```python
from build123d import *

# Parameters (mm, degrees)
SKETCH_1_W        = 30
SKETCH_1_H        = 30
SKETCH_1_W_2      = 26
SKETCH_1_H_2      = 26
EXTRUDE_1_DEPTH   = 270
EXTRUDE_1_2_DEPTH = 270
EXTRUDE_1_3_DEPTH = 270
EXTRUDE_1_4_DEPTH = 270
EXTRUDE_1_5_DEPTH = 270
EXTRUDE_1_6_DEPTH = 270
SKETCH_1_4_W      = 400
SKETCH_1_4_H      = 355
EXTRUDE_2_DEPTH   = 2
SKETCH_3_W        = 25
SKETCH_3_H        = 25
SKETCH_3_W_2      = 22
SKETCH_3_H_2      = 22
EXTRUDE_3_DEPTH   = 200
SKETCH_9_W        = 30
SKETCH_9_H        = 30
EXTRUDE_4_DEPTH   = 290
SKETCH_10_W       = 30
SKETCH_10_H       = 30
EXTRUDE_5_DEPTH   = 330


with BuildPart() as part:
    # Sketch 1 → Extrude 1 (new body)
    with BuildSketch(Plane.XY):
        with Locations((-139.865693992, 17.660065035)):
            Rectangle(SKETCH_1_W, SKETCH_1_H)
        with Locations((-139.865693992, 17.660065035)):
            Rectangle(SKETCH_1_W_2, SKETCH_1_H_2, mode=Mode.SUBTRACT)
    extrude(amount=EXTRUDE_1_DEPTH)



with BuildPart() as body_2:
    # Sketch 1 → Extrude 1 2 (new body)
    with BuildSketch(Plane.XY):
        with Locations((40.134306008, 17.660065035)):
            Rectangle(SKETCH_1_W, SKETCH_1_H)
        with Locations((40.134306008, 17.660065035)):
            Rectangle(SKETCH_1_W_2, SKETCH_1_H_2, mode=Mode.SUBTRACT)
    extrude(amount=EXTRUDE_1_2_DEPTH)


with BuildPart() as body_3:
    # Sketch 1 → Extrude 1 3 (new body)
    with BuildSketch(Plane.XY):
        with Locations((220.134306008, 17.660065035)):
            Rectangle(SKETCH_1_W, SKETCH_1_H)
        with Locations((220.134306008, 17.660065035)):
            Rectangle(SKETCH_1_W_2, SKETCH_1_H_2, mode=Mode.SUBTRACT)
    extrude(amount=EXTRUDE_1_3_DEPTH)


with BuildPart() as body_4:
    # Sketch 1 → Extrude 1 4 (new body)
    with BuildSketch(Plane.XY):
        with Locations((-139.865693992, -297.339934965)):
            Rectangle(SKETCH_1_W, SKETCH_1_H)
        with Locations((-139.865693992, -297.339934965)):
            Rectangle(SKETCH_1_W_2, SKETCH_1_H_2, mode=Mode.SUBTRACT)
    extrude(amount=EXTRUDE_1_4_DEPTH)


with BuildPart() as body_5:
    # Sketch 1 → Extrude 1 5 (new body)
    with BuildSketch(Plane.XY):
        with Locations((40.134306008, -297.339934965)):
            Rectangle(SKETCH_1_W, SKETCH_1_H)
        with Locations((40.134306008, -297.339934965)):
            Rectangle(SKETCH_1_W_2, SKETCH_1_H_2, mode=Mode.SUBTRACT)
    extrude(amount=EXTRUDE_1_5_DEPTH)


with BuildPart() as body_6:
    # Sketch 1 → Extrude 1 6 (new body)
    with BuildSketch(Plane.XY):
        with Locations((220.134306008, -297.339934965)):
            Rectangle(SKETCH_1_W, SKETCH_1_H)
        with Locations((220.134306008, -297.339934965)):
            Rectangle(SKETCH_1_W_2, SKETCH_1_H_2, mode=Mode.SUBTRACT)
    extrude(amount=EXTRUDE_1_6_DEPTH)


with BuildPart() as part_1:
    add(part.part)

    add(body_2.part)  # Extrude 2 merges body 2

    add(body_3.part)  # Extrude 2 merges body 3

    add(body_4.part)  # Extrude 2 merges body 4

    add(body_5.part)  # Extrude 2 merges body 5

    add(body_6.part)  # Extrude 2 merges body 6
    # Sketch 1_4 → Extrude 2 (add)
    with BuildSketch(Plane.XY):
        with Locations((40.134306008, -139.839934965)):
            Rectangle(SKETCH_1_4_W, SKETCH_1_4_H)
    extrude(amount=-EXTRUDE_2_DEPTH)

    # Sketch 3 → Extrude 3 (add)
    with BuildSketch(Plane(origin=(0, 0, -2), x_dir=(-1, 0, 0), z_dir=(0, 0, -1))):
        with Locations((-170.134306008, -9.839934965)):
            Rectangle(SKETCH_3_W, SKETCH_3_H)
        with Locations((-170.134306008, -9.839934965)):
            Rectangle(SKETCH_3_W_2, SKETCH_3_H_2, mode=Mode.SUBTRACT)
        with Locations((-170.134306008, -269.839934965)):
            Rectangle(SKETCH_3_W, SKETCH_3_H)
        with Locations((-170.134306008, -269.839934965)):
            Rectangle(SKETCH_3_W_2, SKETCH_3_H_2, mode=Mode.SUBTRACT)
        with Locations((89.865693992, -269.839934965)):
            Rectangle(SKETCH_3_W, SKETCH_3_H)
        with Locations((89.865693992, -269.839934965)):
            Rectangle(SKETCH_3_W_2, SKETCH_3_H_2, mode=Mode.SUBTRACT)
        with Locations((89.865693992, -9.839934965)):
            Rectangle(SKETCH_3_W, SKETCH_3_H)
        with Locations((89.865693992, -9.839934965)):
            Rectangle(SKETCH_3_W_2, SKETCH_3_H_2, mode=Mode.SUBTRACT)
    extrude(amount=EXTRUDE_3_DEPTH)

    # Sketch 9 → Extrude 4 (add)
    with BuildSketch(Plane(origin=(0, -282.339934965, 0), x_dir=(1, 0, 0), z_dir=(0, 1, 0))):
        with Locations((220.134306008, -15)):
            Rectangle(SKETCH_9_W, SKETCH_9_H)
    extrude_4 = extrude(amount=EXTRUDE_4_DEPTH)

    # Mirror 1: Extrude 4 across plane
    add(extrude_4.mirror(Plane.ZY.offset(-40.134306008)))

    # Sketch 10 → Extrude 5 (add)
    with BuildSketch(Plane.ZY.offset(-205.134306008)):
        with Locations((15, -297.339934965)):
            Rectangle(SKETCH_10_W, SKETCH_10_H)
        with Locations((15, 17.660065035)):
            Rectangle(SKETCH_10_W, SKETCH_10_H)
    extrude(amount=EXTRUDE_5_DEPTH)


solid = part_1.part
```
Input: part model. Units: mm. Frame: model coordinates. A direction names the side the tool comes from. Round coordinates to 2 decimals unless told otherwise and drop trailing zeros. Order: outer loops, then holes, each group sorted by start corner. A loop starts at its lowest first (then second) coordinate and runs counter-clockwise, first axis right, second up. Notation, with made-up numbers: (-16, -22.75) - (4, -22.75) arc R33 ccw to (4, 15.25) - close; hole circle Ø7 at (-9.75, 43.5). An arc over 180 degrees is marked (long way). Answer in a Markdown table with one row per item.
Item 1: Section query C-C (x = -133). Return the cut outline in (y, z).
Model answer:
| item | result |
|---|---|
| outline | (-317.34, -2) - (37.66, -2) - (37.66, 0) - (32.66, 0) - (32.66, 270) - (30.66, 270) - (30.66, 0) - (7.66, 0) - (7.66, 30) - (4.66, 30) - (4.66, 270) - (2.66, 270) - (2.66, 30) - (-282.34, 30) - (-282.34, 270) - (-284.34, 270) - (-284.34, 0) - (-310.34, 0) - (-310.34, 270) - (-312.34, 270) - (-312.34, 0) - (-317.34, 0) - close |
Item 2: Section query B-B (y = -129). Return the cut outline in (x, z).
Model answer:
| item | result |
|---|---|
| outline | (-159.87, -2) - (240.13, -2) - (240.13, 0) - (235.13, 0) - (235.13, 30) - (205.13, 30) - (205.13, 0) - (-124.87, 0) - (-124.87, 30) - (-154.87, 30) - (-154.87, 0) - (-159.87, 0) - close |
Item 3: Mould query, pull axis X, two halves, no side actions, for faces 1 (the flat face through (181.3, -269.8, -202)), 2 (the flat face through (181.134, -270, -101)), 3 (the flat face through (182.634, -10, -101)). Classes: released by +X, released by -X, zero draft, split by the parting line, or undercut.
Model answer:
| item | result |
|---|---|
| face 1 | zero draft |
| face 2 | undercut |
| face 3 | released by +X |
Item 4: Pin query (flat end, axial travel): pin 1 (8 mm diameter, centred on x = -145.5, z = 130, fed in from +Y); pin 2 (21 mm diameter, centred on y = 21.5, z = 122, fed in from +X); pin 3 (2.5 mm diameter, centred on x = 217, y = 6, fed in from +Z). Return the tip coordinate at first contact, or that it passes through.
Model answer:
| item | result |
|---|---|
| pin 1 | stops at y = 32.66 |
| pin 2 | stops at x = 235.13 |
| pin 3 | stops at z = 30 |
Item 5: Reachability of faces 4 (the flat face through (53.134, 17, 148)), 5 (the flat face through (-49, 17, 30)), 6 (the flat face through (-90, 2.66, -101)) from +Z, -Z, +X, -X, +Y, -Y: full face, straight path, thin tool, end or side. Return the list, or none.
Model answer:
| item | result |
|---|---|
| face 4 | +Z |
| face 5 | +Z, +Y, -Y |
| face 6 | -Z, +X, -X, +Y |
Item 6: Section query A-A (z = -44.5). Give the number of separate pieces and of enclosed holes in the cut face, then the cut area to 3 significant figures.
Model answer:
| item | result |
|---|---|
| separate pieces | 4 |
| enclosed holes | 4 |
| area | 564 mm² |
Item 7: Line query: line 1 (X direction, y = -285, z = 46); line 2 (X direction, y = -260, z = -23); line 3 (Z direction, x = 48, y = -34). Output: solid intervals per line, ascending.
Model answer:
| item | result |
|---|---|
| line 1 | x = -154.87 to -152.87, -126.87 to -124.87, 25.13 to 27.13, 53.13 to 55.13, 205.13 to 207.13, 233.13 to 235.13 |
| line 2 | x = -102.37 to -100.87, -78.87 to -77.37, 157.63 to 159.13, 181.13 to 182.63 |
| line 3 | z = -2 to 0 |
